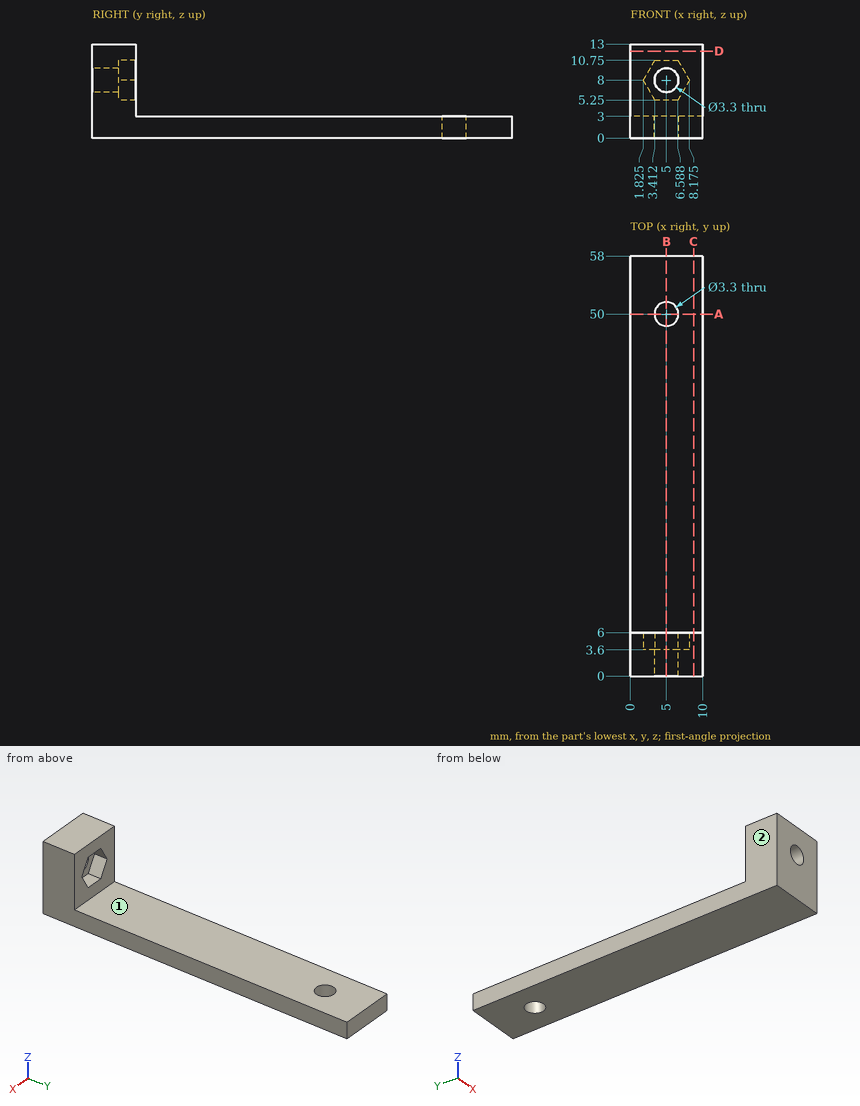
For this review, use the dimensioned drawing (mm, ordinates from the lowest corner) and the shaded views. A direction names the side the tool comes from. Round coordinates to 2 decimals unless told otherwise and drop trailing zeros. Write each loop counter-clockwise with the first axis right and the second up, starting at its lowest first coordinate (ties: lowest second). Pieces come first, ordered by that corner, then holes. Notation, with made-up numbers: (-5.5, -27) -> (40.5, -27) arc R14 ccw to (40.5, -20) -> close; hole circle Ø6 at (1, -3). An arc over 180 degrees is marked (long way). One line per item, written item: value. Start each with the question number.
Q1. Add section C-C (x = 8.75). Give the boundary of the cut face in (y, z), then the cut area to 3 significant figures.
Q2. Insertion check: P1, Ø5, axis at x = 5.5, z = 9.5, coming from the +Y side; P2, Ø2.5, axis at x = 5, z = 8, coming from the +Y side; P3, Ø3, axis at x = 3.5, y = 22, coming from the +Z side. Each pin has a flat end and moves straight along its axis. Give the tip position at first contact, or say it passes through.
Q3. Add section D-D (z = 12). Give the boundary of the cut face in (x, y), then the cut area to 3 significant figures.
Q4. Add section B-B (x = 5). Give the boundary of the cut face in (y, z), then the cut area to 3 significant figures.
Q5. Tool access review of the marked faces 1 and 2: name each direction out of +Z, -Z, +X, -X, +Y, -Y from which nothing blocks a thin tool from reaching the whole face with its end or side.
Q6. To check wall thickness, follow probe 1 along Z at (x, y) = (5, 1.9); probe 2 along X at (y, z) = (1.4, 8); probe 3 along Z at (x, y) = (3.75, 5). State the ranges of each line that lie inside material, in increasing order.
Q7. Add section A-A (y = 50). Give the boundary of the cut face in (x, z).
Response:
1. outline: (0, 0) -> (58, 0) -> (58, 3) -> (6, 3) -> (6, 13) -> (0, 13) -> close
1. area: 234 mm^2
2. P1: stops at y = 6
2. P2: passes through
2. P3: stops at z = 3
3. outline: (0, 0) -> (10, 0) -> (10, 6) -> (0, 6) -> close
3. area: 60.0 mm^2
4. outline: (0, 0) -> (48.35, 0) -> (48.35, 3) -> (6, 3) -> (6, 5.25) -> (3.6, 5.25) -> (3.6, 6.35) -> (0, 6.35) -> close; (0, 9.65) -> (3.6, 9.65) -> (3.6, 10.75) -> (6, 10.75) -> (6, 13) -> (0, 13) -> close; (51.65, 0) -> (58, 0) -> (58, 3) -> (51.65, 3) -> close
4. area: 199 mm^2
5. face 1: +Z, +X, -X, +Y
5. face 2: +Z, -Z, -X, +Y, -Y
6. probe 1: z = 0 to 6.35, 9.65 to 13
6. probe 2: x = 0 to 3.35, 6.65 to 10
6. probe 3: z = 0 to 5.25, 10.75 to 13
7. outline: (0, 0) -> (3.35, 0) -> (3.35, 3) -> (0, 3) -> close; (6.65, 0) -> (10, 0) -> (10, 3) -> (6.65, 3) -> close
